Can you work these out from the model? Positions are in its coordinate system, mm. A direction names the side the tool comes from. Coordinates: 2 decimals unless noted, no trailing zeros. Order: outer loops, then holes, each group sorted by start corner. A loop starts at its lowest first (then second) coordinate and runs counter-clockwise, first axis right, second up. Notation, with made-up numbers: (60.5, 45) -> (65.5, 45) arc R21 ccw to (65.5, 79) -> close; hole circle Ø8 at (-7.75, 51.25). An arc over 180 degrees is marked (long way). Answer in a Markdown table with one row per item.
```python
from build123d import *

# Parameters (mm, degrees)
BOSS_EXTRUDE1_DEPTH = 3
SKETCH2_R           = 1.5
CUT_EXTRUDE1_DEPTH  = 3
SKETCH3_W           = 6.35
SKETCH3_H           = 7.620000001
CUT_EXTRUDE2_DEPTH  = 3
BOSS_EXTRUDE2_DEPTH = 3
FILLET2_R           = 3


with BuildPart() as part:
    # Sketch1 → Boss-Extrude1 (new body)
    with BuildSketch(Plane.XY):
        Polygon((-33.787864348, 18.602457347), (-33.787864348, 14.699262249), (-37.97594504, 14.699262249), (-43.97594504, 20.699262249), (-43.97594504, 28.455124303), (-43.97594504, 70.175124303), (43.97594504, 70.175124303), (43.97594504, 28.455124303), (43.97594504, 20.699262249), (37.97594504, 14.699262249), (33.787864348, 14.699262249), (33.787864348, 18.602457347), align=None)
    extrude(amount=BOSS_EXTRUDE1_DEPTH)

    # Sketch2 → Cut-Extrude1 (cut)
    with BuildSketch(Plane.XY.offset(3)):
        with Locations((37.97594504, 24.699262249)):
            Circle(SKETCH2_R)
        with Locations((37.97594504, 34.699262249)):
            Circle(SKETCH2_R)
        with Locations(Location((-37.97594504, 24.699262249, 0), (0, 0, 180))):
            Circle(SKETCH2_R)
        with Locations(Location((-37.97594504, 34.699262249, 0), (0, 0, 180))):
            Circle(SKETCH2_R)
        with Locations((21.293781262, 61.478152505)):
            Circle(SKETCH2_R)
        with Locations((11.293781262, 61.478152505)):
            Circle(SKETCH2_R)
        with Locations(Location((-11.293781262, 61.478152505, 0), (0, 0, 180))):
            Circle(SKETCH2_R)
        with Locations(Location((-21.293781262, 61.478152505, 0), (0, 0, 180))):
            Circle(SKETCH2_R)
    extrude(amount=-CUT_EXTRUDE1_DEPTH, mode=Mode.SUBTRACT)

    # Sketch3 → Cut-Extrude2 (cut)
    with BuildSketch(Plane(origin=(0, 0, 0), x_dir=(-1, 0, 0), z_dir=(0, 0, -1))):
        with Locations((0.00872995, 61.826506665)):
            Rectangle(SKETCH3_W, SKETCH3_H)
    extrude(amount=-CUT_EXTRUDE2_DEPTH, mode=Mode.SUBTRACT)

    # Sketch4 → Boss-Extrude2 (add)
    with BuildSketch(Plane.XZ.offset(-18.602457347)):
        Polygon((-12.685088164, -20.434120829), (14.947571964, -20.434120829), (14.947571964, -25.434120829), (22.815283287, -25.434120829), (22.815283287, 3), (-22.664716713, 3), (-22.664716713, -25.434120829), (-12.685088164, -25.434120829), align=None)
    extrude(amount=BOSS_EXTRUDE2_DEPTH)

    # Fillet2
    fillet2_edges = [part.edges().sort_by_distance(p)[0] for p in [
        (0.075283287, 15.602457347, 3),
    ]]
    fillet(fillet2_edges, radius=FILLET2_R)


solid = part.part
```
(1) Suppose I cut it at A-A (z = -23). Please give me the cut outline in (x, y), and give its area (3 significant figures).
Response values:
| item | result |
|---|---|
| outline | (-22.66, 15.6) -> (-12.69, 15.6) -> (-12.69, 18.6) -> (-22.66, 18.6) -> close; (14.95, 15.6) -> (22.82, 15.6) -> (22.82, 18.6) -> (14.95, 18.6) -> close |
| area | 53.5 mm2 |
(2) On a 3-axis mill with a long thin cutter (end or side, diameter ignored), from which of +Z, -Z, +X, -X, +Y, -Y can I reach the whole of each face in a straight line? I mean faces 5 (the flat face through (-28, 18.602, 1)), 6 (the flat face through (0, 58.017, 1)), 7 (the flat face through (14.948, 17, -23)). Say none if no direction works.
Response values:
| item | result |
|---|---|
| face 5 | +Z, -Z, -Y |
| face 6 | +Z, -Z |
| face 7 | -Z, +Y, -Y |
(3) Will these pins go through, and if not, where does the flat tip stop? pin 1 Ø0.9 at (x, z) = (-29, 1) entering from -Y; pin 2 Ø2.5 at (x, z) = (-1.5, 2) entering from -Y; pin 3 Ø2.5 at (y, z) = (17, 2) entering from -X; pin 4 Ø1.8 at (x, y) = (-37.98, 24.7) entering from +Z.
Response values:
| item | result |
|---|---|
| pin 1 | y = 18.6 |
| pin 2 | y = 15.7 |
| pin 3 | x = -41.53 |
| pin 4 | through |
(4) I need wall thicknesses on line 1 (Y direction, x = 11, z = -1.25); line 2 (Z direction, x = -17, y = 60); line 3 (X direction, y = 18, z = -2). Which ranges of each line are inside material? Lowest first, please. Write a range as [from, to].
Response values:
| item | result |
|---|---|
| line 1 | [15.6, 18.6] |
| line 2 | [0, 3] |
| line 3 | [-22.66, 22.82] |
(5) Suppose I cut it at C-C (y = 22). Please give me the cut outline in (x, z).
Response values:
| item | result |
|---|---|
| outline | (-43.98, 0) -> (43.98, 0) -> (43.98, 3) -> (-43.98, 3) -> close |
(6) We'd pull the mould along Y, two halves only. Please class faces 1 (the flat face through (-40.934, 17.657, 1.479)), 2 (the flat face through (3.166, 62, 1)), 3 (the flat face through (43.976, 45, 1)), 4 (the flat face through (-1, 70.175, 1)): +Y half, -Y half, draft (parallel to the pull), parting line (faces both ways), or undercut.
Response values:
| item | result |
|---|---|
| face 1 | -Y half |
| face 2 | undercut |
| face 3 | draft |
| face 4 | +Y half |
(7) Suppose I cut it at D-D (z = -8.5). Please give me the cut outline in (x, y).
Response values:
| item | result |
|---|---|
| outline | (-22.66, 15.6) -> (22.82, 15.6) -> (22.82, 18.6) -> (-22.66, 18.6) -> close |
(8) Suppose I cut it at B-B (x = 2). Please give me the cut outline in (y, z).
Response values:
| item | result |
|---|---|
| outline | (15.6, -20.43) -> (18.6, -20.43) -> (18.6, 0) -> (58.02, 0) -> (58.02, 3) -> (18.6, 3) arc R3 ccw to (15.6, 0) -> close; (65.64, 0) -> (70.18, 0) -> (70.18, 3) -> (65.64, 3) -> close |
